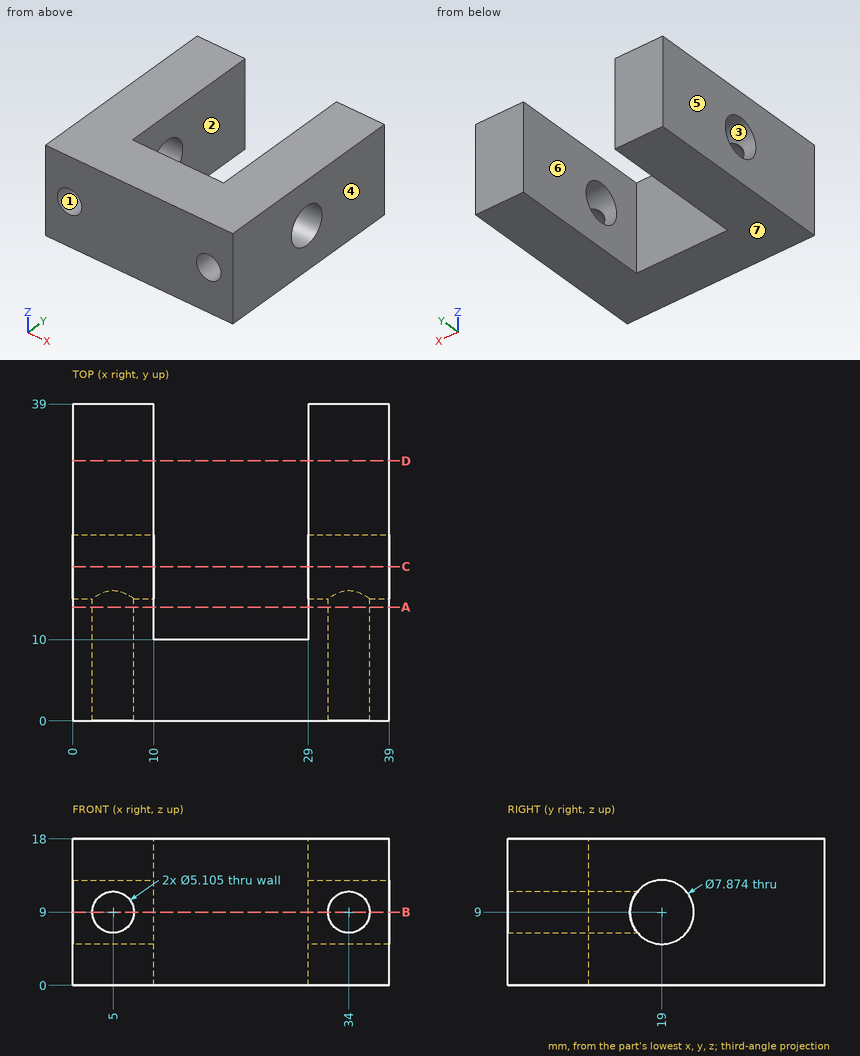
Could you check a few things on this drawing? It's one solid part, dimensions in mm from its lowest x, y, z. A direction names the side the tool comes from. Coordinates: 2 decimals unless noted, no trailing zeros. Order: outer loops, then holes, each group sorted by start corner. A loop starts at its lowest first (then second) coordinate and runs counter-clockwise, first axis right, second up. Notation, with made-up numbers: M 51.5,42.25 L 89.5,42.25 A7 cw 89.5,51.25 Z; hole C 23,-0.75 d1. An arc over 180 degrees is marked long. Answer as CSV lines item,"result".
(1) Suppose I cut it at C-C on y = 19. Please give me the cut outline in (x, z).
Geometry check:
outline,"M 0,0 L 10,0 L 10,5.06 L 0,5.06 Z; M 0,12.94 L 10,12.94 L 10,18 L 0,18 Z; M 29,0 L 39,0 L 39,5.06 L 29,5.06 Z; M 29,12.94 L 39,12.94 L 39,18 L 29,18 Z"
(2) On a 3-axis mill with a long thin cutter (end or side, diameter ignored), from which of +Z, -Z, +X, -X, +Y, -Y can I reach the whole of each face in a straight line? I mean the marked faces 1, 2 and 3. Say none if no direction works.
Geometry check:
face 1,"-Y"
face 2,"+Z, -Z, +Y"
face 3,"+X, -X"
(3) Suppose I cut it at A-A on y = 14. Please give me the cut outline in (x, z) (1 decimal), plus the area to 3 significant figures.
Geometry check:
outline,"M 0,0 L 10,0 L 10,18 L 0,18 Z; M 29,0 L 39,0 L 39,18 L 29,18 Z; hole C 5,9 d5.1; hole C 34,9 d5.1"
area,"319 mm^2"
(4) Suppose I cut it at B-B on z = 9. Please give me the cut outline in (x, y), plus the area to 3 significant figures.
Geometry check:
outline,"M 0,0 L 2.45,0 L 2.45,15.06 L 0,15.06 Z; M 0,22.94 L 10,22.94 L 10,39 L 0,39 Z; M 7.55,0 L 31.45,0 L 31.45,15.06 L 29,15.06 L 29,10 L 10,10 L 10,15.06 L 7.55,15.06 Z; M 29,22.94 L 39,22.94 L 39,39 L 29,39 Z; M 36.55,0 L 39,0 L 39,15.06 L 36.55,15.06 Z"
area,"659 mm^2"
(5) Please list where these lines run through material, in increasing order: L1, parallel to X at y = 9.5, z = 9; L2, parallel to X at y = 11.25, z = 9; L3, parallel to Y at x = 37, z = 9.
Geometry check:
L1,"0 to 2.45, 7.55 to 31.45, 36.55 to 39"
L2,"0 to 2.45, 7.55 to 10, 29 to 31.45, 36.55 to 39"
L3,"0 to 15.06, 22.94 to 39"
(6) If we mould it in two halves opening along X, with no side actions, what happens to the marked faces 4, 5, 6 and 7? For each: released by +X, released by -X, zero draft, split by the parting line, or undercut.
Geometry check:
face 4,"released by +X"
face 5,"released by -X"
face 6,"undercut"
face 7,"zero draft"
(7) I'm going to push flat-ended pins straight in: pin 1 (9 mm diameter, centred on y = 19, z = 9, fed in from +X); pin 2 (3 mm diameter, centred on x = 34, z = 9, fed in from -Y). Where does each tip first touch, or does it pass through?
Geometry check:
pin 1,"x = 39"
pin 2,"y = 22.64"
(8) Suppose I cut it at D-D on y = 32. Please give me the cut outline in (x, z), plus the area to 3 significant figures.
Geometry check:
outline,"M 0,0 L 10,0 L 10,18 L 0,18 Z; M 29,0 L 39,0 L 39,18 L 29,18 Z"
area,"360 mm^2"
